Here's the drawing with two shaded views (mm, measured from the low corner). I have some questions. A direction names the side the tool comes from. Round coordinates to 2 decimals unless told otherwise and drop trailing zeros. Loops run counter-clockwise (first coordinate to the right, second up) from the corner with the lowest first, then second, coordinate; pieces in that order, holes last.
(1) Which directions (+Z, -Z, +X, -X, +Y, -Y) give clear straight access to the entire face, cutting with the end or side of a thin tool? Please do the marked faces 1 and 2.
(2) If I drill on line 1 along Y through (x, z) = (8.5, 8.25); line 2 along X through (y, z) = (3, 5.5), over which ranges is the centre line in solid material (lowest first)?
(3) Thinking about a two-plate mould opening in Y: for the marked faces 3, 4 and 5, which applies, released by +Y, released by -Y, zero draft, split by the parting line, or undercut?
(4) I want a section at A-A on x = 5.5. Write out the boundary of the cut face in (y, z), plus the area to 3 significant figures.
(5) I want a section at D-D on x = 2. Write out the boundary of the cut face in (y, z).
(6) Will these pins go through, and if not, where does the flat tip stop? pin 1 Ø4 at (x, y) = (4, 5) entering from +Z; pin 2 Ø2 at (x, z) = (4, 2) entering from +Y; pin 3 Ø1.5 at (y, z) = (3.5, 8.5) entering from +X.
(7) I want a section at B-B on y = 2.5. Write out the boundary of the cut face in (x, z).
(8) I want a section at C-C on z = 1.25. Write out the boundary of the cut face in (x, y).
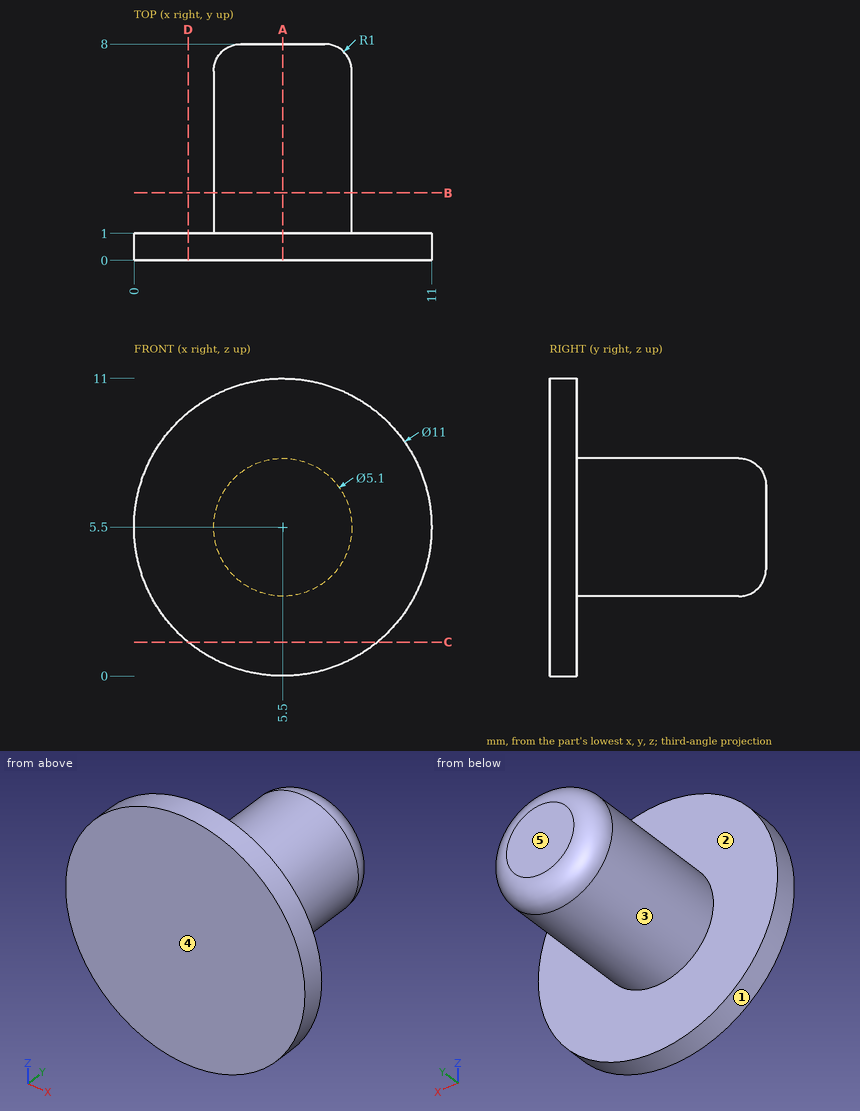
Filled sheet:
1. face 1: +Y, -Y
1. face 2: +Y
2. line 1: y = 0 to 1
2. line 2: x = 2.95 to 8.05
3. face 3: zero draft
3. face 4: released by -Y
3. face 5: released by +Y
4. outline: (0, 0) - (1, 0) - (1, 2.95) - (7, 2.95) arc R1 ccw to (8, 3.95) - (8, 7.05) arc R1 ccw to (7, 8.05) - (1, 8.05) - (1, 11) - (0, 11) - close
4. area: 46.3 mm2
5. outline: (0, 1.26) - (1, 1.26) - (1, 9.74) - (0, 9.74) - close
6. pin 1: stops at z = 8.05
6. pin 2: stops at y = 1
6. pin 3: stops at x = 6.7
7. outline: circle Ø5.1 at (5.5, 5.5)
8. outline: (2.01, 0) - (8.99, 0) - (8.99, 1) - (2.01, 1) - close
